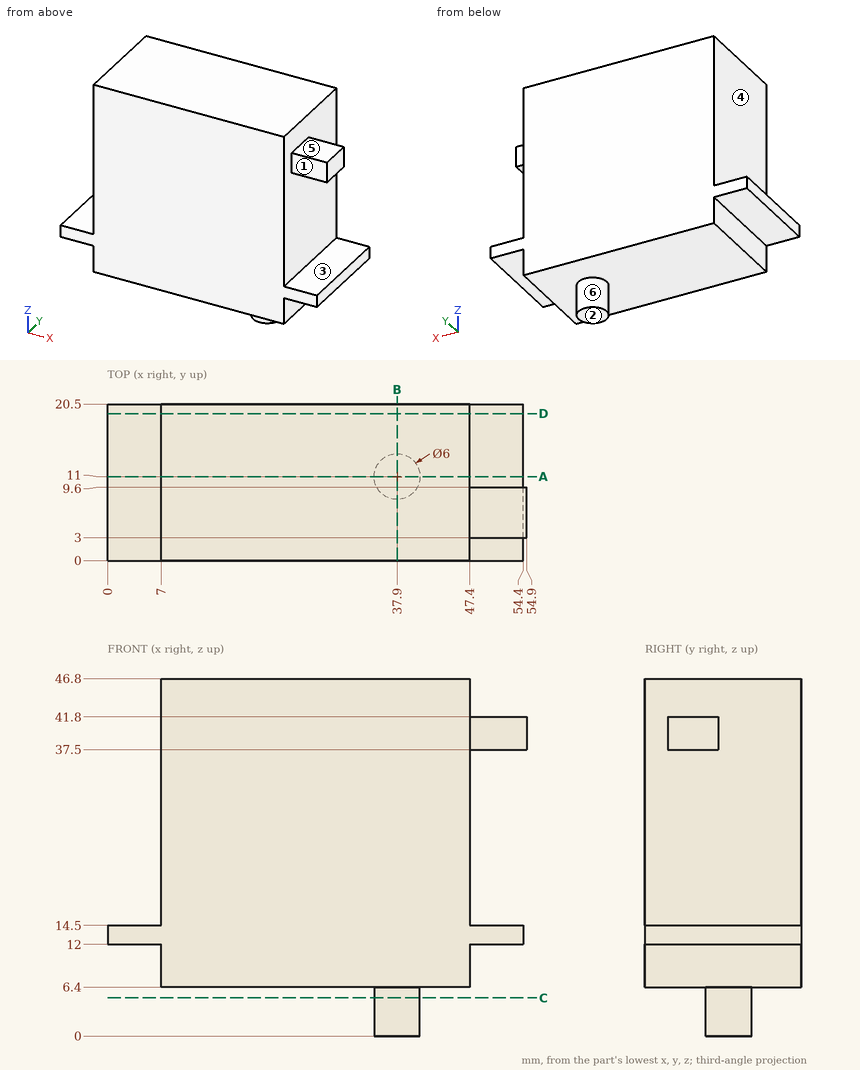
Print and shaded views of the part. All mm, measured from the part's lowest x, y and z. A direction names the side the tool comes from. Give positions to 0.01 mm unless a question says otherwise; leave off trailing zeros. Loops run counter-clockwise (first coordinate to the right, second up) from the corner with the lowest first, then second, coordinate; pieces in that order, holes last. Notation, with made-up numbers: (-32, 38.5) - (7, 38.5) arc R16 ccw to (7, 66.5) - close; hole circle Ø8 at (5, 30.25). An arc over 180 degrees is marked (long way). One line per item, written item: value. Start each with the question number.
1. Slice it at A-A (y = 11). List the corners of the cut face in (x, z), plus the area to 3 significant figures.
2. Pin check, flat tips, straight feed: pin 1 (10 mm diameter, centred on x = 42.5, y = 16, fed in from -Z); pin 2 (5.5 mm diameter, centred on x = 2, y = 9.5, fed in from +Z); pin 3 (4.5 mm diameter, centred on y = 10.5, z = 8, fed in from -X); pin 4 (5 mm diameter, centred on y = 11, z = 5.5, fed in from +X). Stop position of each tip, or through.
3. Slice it at C-C (z = 5). List the corners of the cut face in (x, y).
4. Slice it at B-B (x = 37.9). List the corners of the cut face in (y, z).
5. Probe L1, parallel to X at y = 14.75, z = 28; L2, parallel to Z at x = 32, y = 14.5; L3, parallel to X at y = 5, z = 41. List the from-to ranges inside material, lowest first. Write a range as from..to.
6. Slice it at D-D (y = 19.25). List the corners of the cut face in (x, z).
7. Which spindle directions (+Z, -Z, +X, -X, +Y, -Y) get a long thin tool onto all of the face, cutting with end or side? Do the marked faces 4, 5 and 6. Say none if no direction does.
8. Pull direction Z, two halves, no side cores. Call the marked faces 1, 2 and 3: pulls with the +Z half, pulls with the -Z half, needs draft (parallel to the pull), parting line crosses it, or undercut.
Solution:
1. outline: (0, 12) - (7, 12) - (7, 6.4) - (34.9, 6.4) - (34.9, 0) - (40.9, 0) - (40.9, 6.4) - (47.4, 6.4) - (47.4, 12) - (54.4, 12) - (54.4, 14.5) - (47.4, 14.5) - (47.4, 46.8) - (7, 46.8) - (7, 14.5) - (0, 14.5) - close
1. area: 1,710 mm^2
2. pin 1: stops at z = 0
2. pin 2: stops at z = 14.5
2. pin 3: stops at x = 7
2. pin 4: stops at x = 47.4
3. outline: circle Ø6 at (37.9, 11)
4. outline: (0, 6.4) - (8, 6.4) - (8, 0) - (14, 0) - (14, 6.4) - (20.5, 6.4) - (20.5, 46.8) - (0, 46.8) - close
5. L1: x = 7..47.4
5. L2: z = 6.4..46.8
5. L3: x = 7..54.9
6. outline: (0, 12) - (7, 12) - (7, 6.4) - (47.4, 6.4) - (47.4, 12) - (54.4, 12) - (54.4, 14.5) - (47.4, 14.5) - (47.4, 46.8) - (7, 46.8) - (7, 14.5) - (0, 14.5) - close
7. face 4: +Z, -X, +Y, -Y
7. face 5: +Z, +X, +Y, -Y
7. face 6: -Z
8. face 1: needs draft
8. face 2: pulls with the -Z half
8. face 3: undercut
